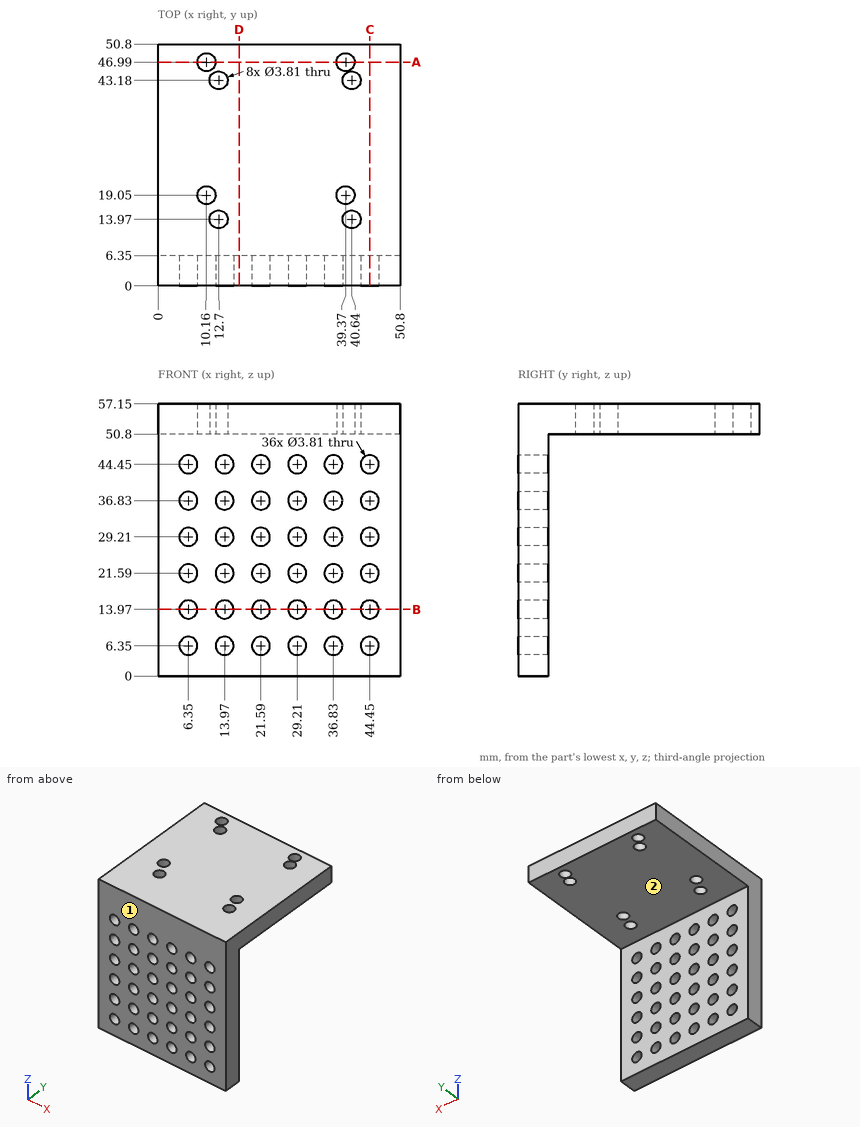
Design review of the part shown in the three views and the two pictorial views. Dimensions are in mm from the part's minimum x, y and z. A direction names the side the tool comes from. Round coordinates to 2 decimals unless told otherwise and drop trailing zeros. Loops run counter-clockwise (first coordinate to the right, second up) from the corner with the lowest first, then second, coordinate; pieces in that order, holes last. Notation, with made-up numbers: (-33, 78.25) - (5, 78.25) arc R35 ccw to (5, 115.25) - close; hole circle Ø11 at (22.5, -20.5). An arc over 180 degrees is marked (long way). Answer as CSV lines item,"result".
(1) Consider section A-A on y = 46.99. Give the boundary of the cut face in (x, z) (3 decimals).
Checked values:
outline,"(0, 50.8) - (8.255, 50.8) - (8.255, 57.15) - (0, 57.15) - close; (12.065, 50.8) - (37.465, 50.8) - (37.465, 57.15) - (12.065, 57.15) - close; (41.275, 50.8) - (50.8, 50.8) - (50.8, 57.15) - (41.275, 57.15) - close"
(2) Tool access review of the marked faces 1 and 2: name each direction out of +Z, -Z, +X, -X, +Y, -Y from which nothing blocks a thin tool from reaching the whole face with its end or side.
Checked values:
face 1,"+Z, -Z, +X, -X, -Y"
face 2,"-Z, +X, -X, +Y"
(3) Wall thickness on line 1 (X direction, y = 19.05, z = 52.75) (3 decimals); line 2 (X direction, y = 46, z = 55); line 3 (Y direction, x = 22.5, z = 48.5): over which ranges is each line inside the solid? List them lowest first.
Checked values:
line 1,"x = 0 to 8.255, 12.065 to 37.465, 41.275 to 50.8"
line 2,"x = 0 to 8.53, 11.79 to 37.74, 41 to 50.8"
line 3,"y = 0 to 6.35"
(4) Insertion check: P1, Ø1.5, axis at x = 23, z = 21.5, coming from the +Y side; P2, Ø6, axis at x = 40.64, y = 43.18, coming from the -Z side. Each pin has a flat end and moves straight along its axis. Give the tip position at first contact, or say it passes through.
Checked values:
P1,"stops at y = 6.35"
P2,"stops at z = 50.8"
(5) Consider section B-B on z = 13.97. Give the boundary of the cut face in (x, y) (3 decimals).
Checked values:
outline,"(0, 0) - (4.445, 0) - (4.445, 6.35) - (0, 6.35) - close; (8.255, 0) - (12.065, 0) - (12.065, 6.35) - (8.255, 6.35) - close; (15.875, 0) - (19.685, 0) - (19.685, 6.35) - (15.875, 6.35) - close; (23.495, 0) - (27.305, 0) - (27.305, 6.35) - (23.495, 6.35) - close; (31.115, 0) - (34.925, 0) - (34.925, 6.35) - (31.115, 6.35) - close; (38.735, 0) - (42.545, 0) - (42.545, 6.35) - (38.735, 6.35) - close; (46.355, 0) - (50.8, 0) - (50.8, 6.35) - (46.355, 6.35) - close"
(6) Consider section D-D on x = 17. Give the boundary of the cut face in (y, z).
Checked values:
outline,"(0, 0) - (6.35, 0) - (6.35, 50.8) - (50.8, 50.8) - (50.8, 57.15) - (0, 57.15) - close"
(7) Consider section C-C on x = 44.45. Give the number of separate pieces and of enclosed holes in the cut face, then the cut area to 3 significant figures.
Checked values:
separate pieces,"7"
enclosed holes,"0"
area,"500 mm2"
